```python
from build123d import *

# Parameters (mm, degrees)
F0_R           = 17.5
F0_R_2         = 5
F1_DEPTH       = 1.5
F2_D           = 5
F2_CSINK_D     = 7
F2_CSINK_ANGLE = 90
F4_R           = 0.7


# Not quite as in the source:
# - a fillet or chamfer that OpenCascade refuses, or shapes differently, is made with other operations: its cross-section is extruded or revolved along the edge and cut away or added


with BuildPart() as f1:
    # F0 (on Front) → F1 (new body)
    with BuildSketch(Plane.XZ):
        Circle(F0_R)
        Circle(F0_R_2, mode=Mode.SUBTRACT)
    extrude(amount=-F1_DEPTH)

    # F2 (through all)
    with Locations(Plane.XZ):
        with Locations((-11.7, 0), (11.7, 0)):
            CounterSinkHole(F2_D / 2, F2_CSINK_D / 2, counter_sink_angle=F2_CSINK_ANGLE)

    # F3: fillet of radius 2 on 1 edges, made by hand

    # F3_s1 → F3_t2 (revolve, cut)
    with BuildSketch(Plane.XY):
        with BuildLine():
            ThreePointArc((17.5, 1.5), (16.7882531983, 0.4188611699), (15.5635083269, 0))
            Line((15.5635083269, 0), (17.5, 0))
            Line((17.5, 0), (17.5, 1.5))
        make_face()
    revolve(axis=Axis((0, 0, 0), (0, -1, 0)), mode=Mode.SUBTRACT)

    # F4
    f4_edges = [f1.edges().sort_by_distance(p)[0] for p in [
        (-5, 0, 0),
        (-5, 1.5, 0),
    ]]
    fillet(f4_edges, radius=F4_R)


solid = f1.part
```
Input: part model. Units: mm. Frame: model coordinates. Round coordinates to 2 decimals unless told otherwise and drop trailing zeros. Loops run counter-clockwise (first coordinate to the right, second up) from the corner with the lowest first, then second, coordinate; pieces in that order, holes last. Notation, with made-up numbers: (56.5, -25.5) -> (61.5, -25.5) arc R22 ccw to (61.5, -6.5) -> close; hole circle Ø3 at (-34, -23.5). An arc over 180 degrees is marked (long way). One line per item, written item: value.
(1) Material intervals for line 1 (Y direction, x = 6, z = 16); line 2 (Z direction, x = -3, y = 0.6); line 3 (X direction, y = 1.05, z = -3), sorted ascending. Write a range as [from, to].
Geometry check:
line 1: [0.71, 1.5]
line 2: [-16.72, -4.01], [4.01, 16.72]
line 3: [-17.06, -4.06], [4.06, 17.06]
(2) Pin query (flat end, axial travel): pin 1 (12 mm diameter, centred on x = 11.5, z = -1.5, fed in from -Y); pin 2 (9 mm diameter, centred on x = 0, z = 0, fed in from +Y); pin 3 (6.5 mm diameter, centred on x = -11.7, z = 0, fed in from -Y). Return the tip coordinate at first contact, or that it passes through.
Geometry check:
pin 1: y = 0
pin 2: through
pin 3: y = 0.25
(3) Mould query, pull axis X, two halves, no side actions, for faces 1 (the face through (0, 1.5, -8)), 2 (the face through (-14.085, 1.254, 0.751)). Classes: pulls with the +X half, pulls with the -X half, needs draft (parallel to the pull), parting line crosses it, or undercut.
Geometry check:
face 1: needs draft
face 2: undercut
(4) Section A-A (z = 0). Return the cut outline in (x, y).
Geometry check:
outline: (-17.5, 1.5) arc R2 ccw to (-15.56, 0) -> (-15.2, 0) -> (-14.2, 1) -> (-14.2, 1.5) -> close; (-9.2, 1) -> (-8.2, 0) -> (-5.7, 0) arc R0.7 ccw to (-5, 0.7) -> (-5, 0.8) arc R0.7 ccw to (-5.7, 1.5) -> (-9.2, 1.5) -> close; (5, 0.7) arc R0.7 ccw to (5.7, 0) -> (8.2, 0) -> (9.2, 1) -> (9.2, 1.5) -> (5.7, 1.5) arc R0.7 ccw to (5, 0.8) -> close; (14.2, 1) -> (15.2, 0) -> (15.56, 0) arc R2 ccw to (17.5, 1.5) -> (14.2, 1.5) -> close
(5) Section B-B (x = 0). Return the cut outline in (y, z).
Geometry check:
outline: (0, -15.56) arc R2 ccw to (1.5, -17.5) -> (1.5, -5.7) arc R0.7 ccw to (0.8, -5) -> (0.7, -5) arc R0.7 ccw to (0, -5.7) -> close; (0, 5.7) arc R0.7 ccw to (0.7, 5) -> (0.8, 5) arc R0.7 ccw to (1.5, 5.7) -> (1.5, 17.5) arc R2 ccw to (0, 15.56) -> close
